```python
from build123d import *

# Parameters (mm, degrees)
F1_DEPTH = 152.4
F2_R     = 1.98374
F3_R     = 3.69316
F4_W     = 9.5329248
F4_H     = 24
F4_R     = 1.35255
F5_DEPTH = 1.70942
F6_R     = 1.35255
F6_R_2   = 1.8288
F7_DEPTH = 1.70942


with BuildPart() as f1:
    # F0 (on Top) → F1 (new body)
    with BuildSketch(Plane.XY):
        Polygon((0, 32.3337428), (0, 0), (-85.6425008, 0), (-85.6425008, 32.3337428), (-87.3519208, 32.3337428), (-87.3519208, -1.70942), (1.70942, -1.70942), (1.70942, 32.3337428), align=None)
    extrude(amount=F1_DEPTH)

    # F2
    f2_edges = [f1.edges().sort_by_distance(p)[0] for p in [
        (0, 0, 76.2),
        (-85.642501, 0, 76.2),
    ]]
    fillet(f2_edges, radius=F2_R)

    # F3
    f3_edges = [f1.edges().sort_by_distance(p)[0] for p in [
        (1.70942, -1.70942, 76.2),
        (-87.351921, -1.70942, 76.2),
    ]]
    fillet(f3_edges, radius=F3_R)

    # F4 (on face) → F5 (cut, through all)
    with BuildSketch(Plane(origin=(0, 0, 0), x_dir=(-1, 0, 0), z_dir=(0, 1, 0))):
        with Locations((74.5712504, 15.175)):
            Rectangle(F4_W, F4_H)
        with Locations((11.0712504, 15.175)):
            Rectangle(F4_W, F4_H)
        with Locations((11.0712504, 137.225)):
            Rectangle(F4_W, F4_H)
        with Locations((74.5712504, 137.225)):
            Rectangle(F4_W, F4_H)
        with Locations((60.20308, 6.35)):
            Circle(F4_R)
        with Locations((25.4394208, 6.35)):
            Circle(F4_R)
        with Locations((25.4394208, 146.05)):
            Circle(F4_R)
        with Locations((60.20308, 146.05)):
            Circle(F4_R)
    extrude(amount=-F5_DEPTH, mode=Mode.SUBTRACT)

    # F6 (on face) → F7 (cut, through all)
    with BuildSketch(Plane.XZ.offset(1.70942)):
        with Locations((-63.1831604, 89.69375)):
            Circle(F6_R)
        with Locations((-22.4593404, 89.69375)):
            Circle(F6_R)
        with Locations((-22.4593404, 62.70625)):
            Circle(F6_R)
        with Locations((-63.1831604, 62.70625)):
            Circle(F6_R)
        with Locations((-50.7587504, 54.76875)):
            Circle(F6_R_2)
        with Locations((-34.8837504, 54.76875)):
            Circle(F6_R_2)
    extrude(amount=-F7_DEPTH, mode=Mode.SUBTRACT)


solid = f1.part
```
Can you work these out from the model? Positions are in its coordinate system, mm. A direction names the side the tool comes from. Round coordinates to 2 decimals unless told otherwise and drop trailing zeros. Loops run counter-clockwise (first coordinate to the right, second up) from the corner with the lowest first, then second, coordinate; pieces in that order, holes last.
Item 1: Please list where these lines run through material, in increasing order: L1, parallel to X at y = 4.5, z = 38.5; L2, parallel to Y at x = -54, z = 100.5.
Item 2: If we mould it in two halves opening along X, with no side actions, what happens to faces 3 (the flat face through (1.709, 17, 75)), 4 (the cylindrical face through (-25.15, -0.84, 144.73)), 5 (the flat face through (-63, -1, 152.4))? For each: +X half, -X half, draft (parallel to the pull), parting line (faces both ways), or undercut.
Item 3: Suppose I cut it at A-A, the plane z = 141.5. Write out the boundary of the cut face in (x, y), then the cut area to 3 significant figures.
Item 4: Suppose I cut it at B-B, the plane y = 3.5. Write out the boundary of the cut face in (x, z).
Item 5: Suppose I cut it at D-D, the plane z = 40.5. Write out the boundary of the cut face in (x, y), then the cut area to 3 significant figures.
Item 6: Will these pins go through, and if not, where does the flat tip stop? pin 1 Ø1.9 at (y, z) = (-0.5, 138) entering from -X; pin 2 Ø4.5 at (x, z) = (-25.44, 146.05) entering from +Y; pin 3 Ø1.6 at (x, z) = (-22.46, 62.71) entering from -Y; pin 4 Ø1.4 at (y, z) = (-1, 14) entering from +X.
Item 7: Which directions (+Z, -Z, +X, -X, +Y, -Y) give clear straight access to the entire face, cutting with the end or side of a thin tool? Please do faces 1 (the flat face through (-42, 0, 75)), 2 (the flat face through (-87.352, 17, 75)).
Item 8: Suppose I cut it at C-C, the plane x = -76.5. Write out the boundary of the cut face in (y, z) (3 decimals), then the cut area to 3 significant figures.
Reported:
1. L1: x = -87.35 to -85.64, 0 to 1.71
1. L2: y = -1.71 to 0
2. face 3: +X half
2. face 4: undercut
2. face 5: draft
3. outline: (-87.35, 1.98) arc R3.69 ccw to (-83.66, -1.71) - (-79.34, -1.71) - (-79.34, 0) - (-83.66, 0) arc R1.98 cw to (-85.64, 1.98) - (-85.64, 32.33) - (-87.35, 32.33) - close; (-69.8, -1.71) - (-15.84, -1.71) - (-15.84, 0) - (-69.8, 0) - close; (-6.3, -1.71) - (-1.98, -1.71) arc R3.69 ccw to (1.71, 1.98) - (1.71, 32.33) - (0, 32.33) - (0, 1.98) arc R1.98 cw to (-1.98, 0) - (-6.3, 0) - close
3. area: 226 mm2
4. outline: (-87.35, 0) - (-85.64, 0) - (-85.64, 152.4) - (-87.35, 152.4) - close; (0, 0) - (1.71, 0) - (1.71, 152.4) - (0, 152.4) - close
5. outline: (-87.35, 1.98) arc R3.69 ccw to (-83.66, -1.71) - (-1.98, -1.71) arc R3.69 ccw to (1.71, 1.98) - (1.71, 32.33) - (0, 32.33) - (0, 1.98) arc R1.98 cw to (-1.98, 0) - (-83.66, 0) arc R1.98 cw to (-85.64, 1.98) - (-85.64, 32.33) - (-87.35, 32.33) - close
5. area: 259 mm2
6. pin 1: stops at x = -87.02
6. pin 2: stops at y = 0
6. pin 3: passes through
6. pin 4: stops at x = 0.92
7. face 1: +Z, -Z, +Y
7. face 2: +Z, -Z, -X, +Y, -Y
8. outline: (-1.709, 0) - (0, 0) - (0, 3.175) - (-1.709, 3.175) - close; (-1.709, 27.175) - (0, 27.175) - (0, 125.225) - (-1.709, 125.225) - close; (-1.709, 149.225) - (0, 149.225) - (0, 152.4) - (-1.709, 152.4) - close
8. area: 178 mm2
